Here's how the part is built. I have some questions about the finished solid (model axes, mm). Face numbers are marked on the shaded views. Coordinates: 2 decimals unless noted, no trailing zeros. Write each loop counter-clockwise with the first axis right and the second up, starting at its lowest first coordinate (ties: lowest second). Pieces come first, ordered by that corner, then holes.
```python
from build123d import *


with BuildPart() as part:
    # Sketch → Revolution (revolve)
    with BuildSketch(Plane.XZ):
        with BuildLine():
            Line((0, 82.364962), (-27.55722, 82.364962))
            Line((-27.55722, 82.364962), (-26.5, 91.364962))
            Line((-26.5, 91.364962), (-27.5, 91.364962))
            Line((-27.5, 91.364962), (-38, 1.97956))
            ThreePointArc((-38, 1.97956), (-38.895285, 0.377621), (-37.129481, 0.877301))
            Line((-37.129481, 0.877301), (-27.674688, 81.364962))
            Line((-27.674688, 81.364962), (0, 81.364962))
            Line((0, 81.364962), (0, 82.364962))
        make_face()
    revolve(axis=Axis((0, 0, 0), (0, 0, 1)))


solid = part.part
```
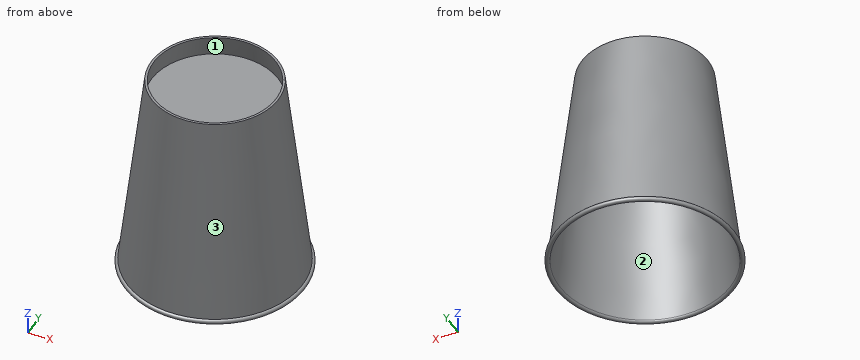
1) Imagine slicing it at C-C on z = 49.5. Please give me the cut outline in (x, y), then the cut area to 3 significant figures.
Values follow:
outline: circle Ø64.84 at (0, 0); hole circle Ø62.84 at (0, 0)
area: 201 mm2
2) Imagine slicing it at A-A on y = 0. Please give me the cut outline in (x, z).
Values follow:
outline: (-38, 1.98) arc R0.99 ccw (long way) to (-37.13, 0.88) - (-27.67, 81.36) - (27.67, 81.36) - (37.13, 0.88) arc R0.99 ccw (long way) to (38, 1.98) - (27.5, 91.36) - (26.5, 91.36) - (27.56, 82.36) - (-27.56, 82.36) - (-26.5, 91.36) - (-27.5, 91.36) - close
3) Imagine slicing it at D-D on z = 10.5. Please give me the cut outline in (x, y), then the cut area to 3 significant figures.
Values follow:
outline: circle Ø74 at (0, 0); hole circle Ø72 at (0, 0)
area: 229 mm2
4) I need wall thicknesses on probe 1 along Y at (x, z) = (20.5, 71); probe 2 along Z at (x, y) = (-14, -20); probe 3 along Y at (x, z) = (-26, 6.5). Which ranges of each line are inside material? Lowest first, please.
Values follow:
probe 1: y = -21.76 to -20.36, 20.36 to 21.76
probe 2: z = 81.36 to 82.36
probe 3: y = -26.98 to -25.57, 25.57 to 26.98
5) We'd pull the mould along Y, two halves only. Please class the marked faces 1, 2 and 3: pulls with the +Y half, pulls with the -Y half, needs draft (parallel to the pull), parting line crosses it, or undercut.
Values follow:
face 1: undercut
face 2: undercut
face 3: parting line crosses it
6) Will these pins go through, and if not, where does the flat tip stop? pin 1 (3 mm diameter, centred on y = 10.5, z = 61.5, fed in from +X); pin 2 (1.5 mm diameter, centred on y = -28, z = 29.5, fed in from -X); pin 3 (4 mm diameter, centred on x = -18.5, z = 63, fed in from -Y); pin 4 (8 mm diameter, centred on x = -23.5, y = -19, fed in from +Z).
Values follow:
pin 1: stops at x = 29.71
pin 2: stops at x = -21.6
pin 3: stops at y = -26.08
pin 4: stops at z = 91.36
